The model under review builds one solid part; all positions refer to its coordinate system, in mm. Face numbers are marked on the shaded views. Coordinates: 2 decimals unless noted, no trailing zeros. Loops run counter-clockwise (first coordinate to the right, second up) from the corner with the lowest first, then second, coordinate; pieces in that order, holes last. Notation, with made-up numbers: M 10.25,36 L 60.25,36 A15 cw 60.25,55 Z; hole C -9.75,9 d6. An arc over 180 degrees is marked long. Use one line per item in the form item = value.
```python
from build123d import *

# Parameters (mm, degrees)
SKETCH_1_R      = 3
EXTRUDE_1_DEPTH = 1.6
CHAMFER_1_SIZE  = 1.6
SKETCH_2_R      = 1.4
EXTRUDE_2_DEPTH = 18.4
CHAMFER_2_SIZE  = 0.2


with BuildPart() as part:
    # 草图1 → 凸台-拉伸1 (new body)
    with BuildSketch(Plane(origin=(0, 0, 0), x_dir=(1, 0, 0), z_dir=(0, 1, 0))):
        with Locations(Location((0, 0, 0), (0, 0, 270))):
            Circle(SKETCH_1_R)
        Polygon((0, -1.154700538), (1, -0.577350269), (1, 0.577350269), (0, 1.154700538), (-1, 0.577350269), (-1, -0.577350269), align=None, mode=Mode.SUBTRACT)
    extrude(amount=EXTRUDE_1_DEPTH)

    # 倒角1
    # the kernel refuses this chamfer: 1.6 mm, written as the material it takes off along each edge
    with BuildSketch(Plane(origin=(0, 1.6, 0), x_dir=(0, 0, 1), z_dir=(-1, 0, 0))) as chamfer_1_piece_1:
        Polygon((3, -CHAMFER_1_SIZE), (3 - CHAMFER_1_SIZE, 0), (3, 0), align=None)
    revolve(axis=Axis((0, 1.6, 0), (0, 1, 0)), mode=Mode.SUBTRACT)

    # 草图2 → 凸台-拉伸2 (add)
    with BuildSketch(Plane(origin=(0, 1.6, 0), x_dir=(1, 0, 0), z_dir=(0, 1, 0))):
        with Locations(Location((0, 0, 0), (0, 0, 270))):
            Circle(SKETCH_2_R)
    extrude(amount=EXTRUDE_2_DEPTH)

    # 倒角2
    chamfer_2_edges = [part.edges().sort_by_distance(p)[0] for p in [
        (0, 20, -1.4),
    ]]
    chamfer(chamfer_2_edges, length=CHAMFER_2_SIZE)


solid = part.part
```
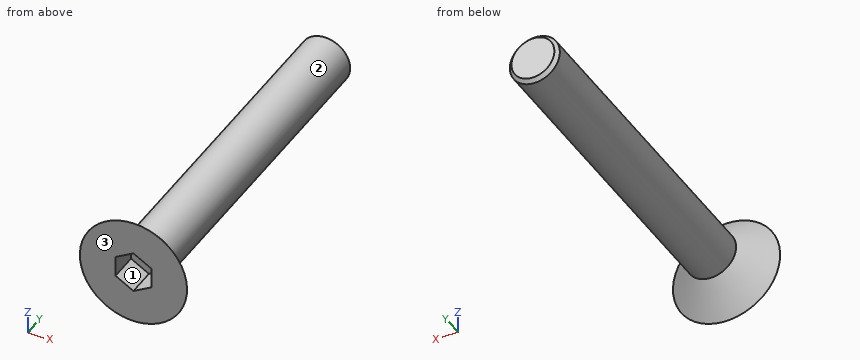
1. Add section B-B (y = 3.5). State the section outline as (x, z) points, then the cut area to 3 significant figures.
Response values:
outline = C 0,0 d2.8
area = 6.16 mm^2
2. The part is to be moulded in two halves that separate along Z. For the marked faces 1, 2 and 3, say which applies: pulls with the +Z half, pulls with the -Z half, needs draft (parallel to the pull), parting line crosses it, or undercut.
Response values:
face_1 = undercut
face_2 = parting line crosses it
face_3 = needs draft
3. Add section A-A (z = 0). State the section outline as (x, y) points, then the cut area to 3 significant figures.
Response values:
outline = M -3,0 L -1,0 L -1,1.6 L 1,1.6 L 1,0 L 3,0 L 1.4,1.6 L 1.4,19.8 L 1.2,20 L -1.2,20 L -1.4,19.8 L -1.4,1.6 Z
area = 55.3 mm^2
4. Insertion check: P1, Ø3, axis at x = 1, y = 8, coming from the -Z side; P2, Ø1.3, axis at y = 1, z = 0, coming from the +X side; P3, Ø1, axis at x = 1.5, y = 12, coming from the +Z side. Each pin has a flat end and moves straight along its axis. Give the tip position at first contact, or say it passes through.
Response values:
P1 = -1.4
P2 = 2.65
P3 = 0.98
5. Wall thickness on line 1 along Y through (x, z) = (0.5, -0.2); line 2 along Y through (x, z) = (-1.6, 1.2); line 3 along X through (y, z) = (17.75, 0.1): over which ranges is each line inside the solid? List them lowest first. Write a range as from..to.
Response values:
line_1 = 1.6..20
line_2 = 0..1
line_3 = -1.4..1.4
